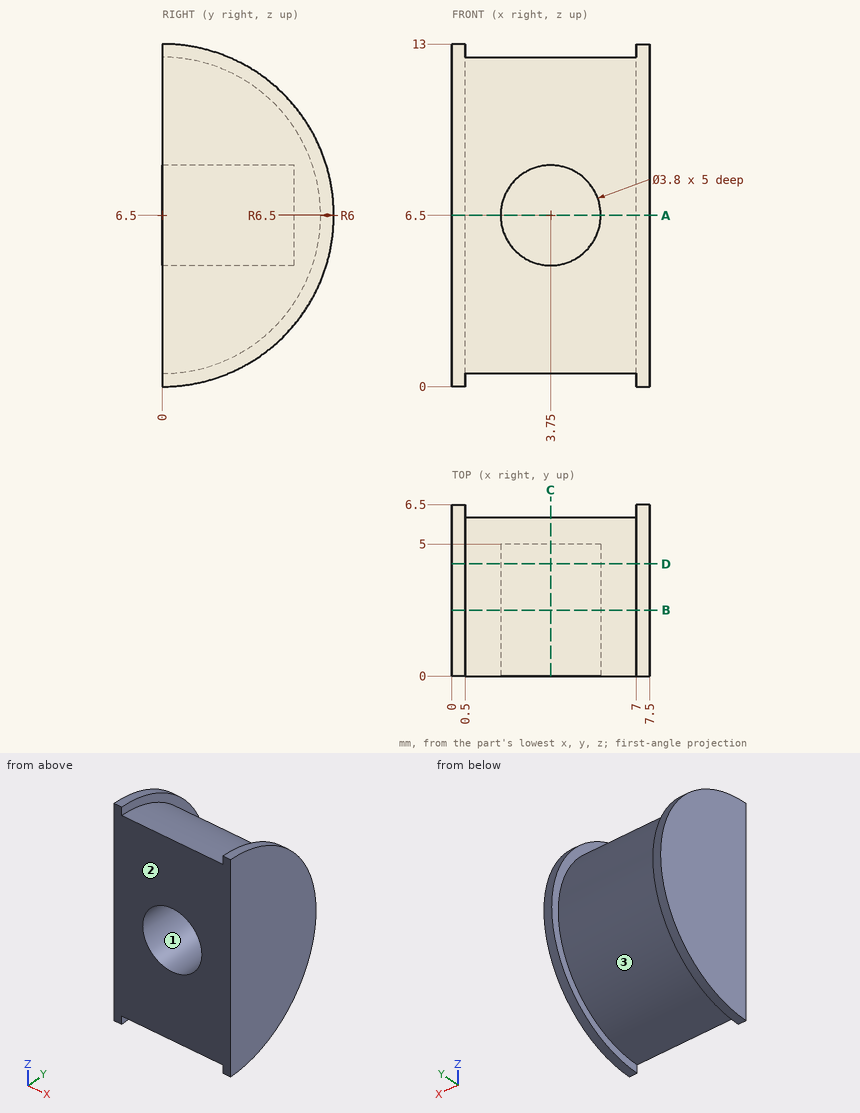
Part print with two shaded views. Sizes in mm from the minimum x, y, z corner. Round coordinates to 2 decimals unless told otherwise and drop trailing zeros. Order: outer loops, then holes, each group sorted by start corner. A loop starts at its lowest first (then second) coordinate and runs counter-clockwise, first axis right, second up. Notation, with made-up numbers: M -30,-37.75 L -11,-37.75 A17 cw -11,-6.75 Z; hole C -9.5,40.5 d7. An arc over 180 degrees is marked long. Use CSV: the item, a comma, the result in double quotes.
Item 1: Pin check, flat tips, straight feed: pin 1 (1 mm diameter, centred on x = 4.5, y = 5.5, fed in from -Z); pin 2 (2.5 mm diameter, centred on x = 3.75, z = 6.5, fed in from +Y). Stop position of each tip, or through.
Worked answers:
pin 1,"z = 3.18"
pin 2,"y = 6"
Item 2: Probe probe 1 along X at (y, z) = (3.25, 6.5); probe 2 along Z at (x, y) = (2.5, 1); probe 3 along X at (y, z) = (4, 5.25). List the from-to ranges inside material, lowest first.
Worked answers:
probe 1,"0 to 1.85, 5.65 to 7.5"
probe 2,"0.58 to 5.07, 7.93 to 12.42"
probe 3,"0 to 2.32, 5.18 to 7.5"
Item 3: Saw through at A-A (z = 6.5). List the corners of the cut face in (x, y).
Worked answers:
outline,"M 0,0 L 1.85,0 L 1.85,5 L 5.65,5 L 5.65,0 L 7.5,0 L 7.5,6.5 L 7,6.5 L 7,6 L 0.5,6 L 0.5,6.5 L 0,6.5 Z"
Item 4: Saw through at B-B (y = 2.5). List the corners of the cut face in (x, z).
Worked answers:
outline,"M 0,0.5 L 0.5,0.5 L 0.5,1.05 L 7,1.05 L 7,0.5 L 7.5,0.5 L 7.5,12.5 L 7,12.5 L 7,11.95 L 0.5,11.95 L 0.5,12.5 L 0,12.5 Z; hole C 3.75,6.5 d3.8"
Item 5: Saw through at C-C (x = 3.75). List the corners of the cut face in (y, z).
Worked answers:
outline,"M 0,0.5 A6 ccw 0,12.5 L 0,8.4 L 5,8.4 L 5,4.6 L 0,4.6 Z"
Item 6: Saw through at D-D (y = 4.25). List the corners of the cut face in (x, z), plus the area to 3 significant figures.
Worked answers:
outline,"M 0,1.58 L 0.5,1.58 L 0.5,2.26 L 7,2.26 L 7,1.58 L 7.5,1.58 L 7.5,11.42 L 7,11.42 L 7,10.74 L 0.5,10.74 L 0.5,11.42 L 0,11.42 Z; hole C 3.75,6.5 d3.8"
area,"53.6 mm²"
Item 7: Pull direction Z, two halves, no side cores. Call the marked faces 1, 2 and 3: released by +Z, released by -Z, zero draft, split by the parting line, or undercut.
Worked answers:
face 1,"undercut"
face 2,"zero draft"
face 3,"split by the parting line"
